Geometry: final body of the model. Coordinates: model frame, mm. A direction names the side the tool comes from. Give positions to 0.01 mm unless a question says otherwise; leave off trailing zeros. Loops run counter-clockwise (first coordinate to the right, second up) from the corner with the lowest first, then second, coordinate; pieces in that order, holes last.
1. Material intervals for line 1 along X through (y, z) = (-7.1, 8); line 2 along X through (y, z) = (-4.75, 2.5); line 3 along Z through (x, y) = (51, -8.35), sorted ascending.
2. Draft query along X for faces 4 (the face through (62, -5, 6)), 5 (the face through (12.66, -7.97, 9.52)), 6 (the face through (0, -5, 7)), 7 (the face through (31, -10, 8)). Return one class per face: +X half, -X half, draft (parallel to the pull), parting line (faces both ways), or undercut.
3. First-contact query: P1, Ø1, axis at x = 30.5, y = -1, coming from the -Z side; P2, Ø4, axis at x = 11, z = 8, coming from the -Y side. Flat tips, straight axial feed; report the tip coordinate or a pass-through.
4. Section A-A, the plane x = 20. Output: boundary loops of the cut face in (y, z).
5. Access query for faces 1 (the face through (2, -5, 0)), 2 (the face through (53.248, -7.972, 8.099)), 3 (the face through (57, -5, 2)). Directions: +Z, -Z, +X, -X, +Y, -Y. A direction counts if a zero-diameter tool reaches every point of the face in a straight line with its end or side. Return the directions, or none.
from build123d import *

# Parameters (mm, degrees)
F1_DEPTH = 10
F3_D     = 4.5
F3_DEPTH = 4
F3_TIP   = 1.3519363928


with BuildPart() as f1:
    # F0 (on Front) → F1 (new body)
    with BuildSketch(Plane.XZ):
        Polygon((0, 13), (0, 0), (5, 0), (5, 4), (57, 4), (57, 0), (62, 0), (62, 13), align=None)
    extrude(amount=F1_DEPTH)

    # F3
    with Locations(Plane.XZ.offset(10)):
        with Locations((11, 8), (51, 8)):
            Hole(F3_D / 2, depth=F3_DEPTH)
            with Locations((0, 0, -(F3_DEPTH + F3_TIP / 2))):  # 118° drill point
                Cone(0, F3_D / 2, F3_TIP, mode=Mode.SUBTRACT)


solid = f1.part
Answers below:
1. line 1: x = 0 to 8.75, 13.25 to 48.75, 53.25 to 62
1. line 2: x = 0 to 5, 57 to 62
1. line 3: z = 4 to 5.75, 10.25 to 13
2. face 4: +X half
2. face 5: undercut
2. face 6: -X half
2. face 7: draft
3. P1: stops at z = 4
3. P2: stops at y = -5.85
4. outline: (-10, 4) - (0, 4) - (0, 13) - (-10, 13) - close
5. face 1: -Z, +X, -X, +Y, -Y
5. face 2: -Y
5. face 3: -Z, +Y, -Y
